```python
from build123d import *

# Parameters (mm, degrees)
BOSS_EXTRUDE1_DEPTH = 2
BOSS_EXTRUDE2_DEPTH = 19
SKETCH6_R           = 1.5
CUT_EXTRUDE1_DEPTH  = 221.788733523


with BuildPart() as part:
    # Sketch1 → Boss-Extrude1 (new body)
    with BuildSketch(Plane.XY):
        Polygon((12.5, -110.17766953), (-12.5, -110.17766953), (-30.17766953, -92.5), (-129.82233047, -92.5), (-147.5, -110.17766953), (-172.5, -110.17766953), (-190.17766953, -92.5), (-190.17766953, -67.5), (-172.5, -49.82233047), (-172.5, 49.82233047), (-190.17766953, 67.5), (-190.17766953, 92.5), (-172.5, 110.17766953), (-147.5, 110.17766953), (-129.82233047, 92.5), (-30.17766953, 92.5), (-12.5, 110.17766953), (12.5, 110.17766953), (30.17766953, 92.5), (30.17766953, 67.5), (12.5, 49.82233047), (12.5, -49.82233047), (30.17766953, -67.5), (30.17766953, -92.5), align=None)
        Polygon((-30.17766953, -67.5), (-12.5, -49.82233047), (-12.5, 49.82233047), (-30.17766953, 67.5), (-129.82233047, 67.5), (-147.5, 49.82233047), (-147.5, -49.82233047), (-129.82233047, -67.5), align=None, mode=Mode.SUBTRACT)
    extrude(amount=BOSS_EXTRUDE1_DEPTH)

    # Sketch2 → Boss-Extrude2 (add)
    with BuildSketch(Plane(origin=(0, 0, 0), x_dir=(-1, 0, 0), z_dir=(0, 0, -1))):
        Polygon((30.17766953, -67.5), (12.5, -67.5), (12.5, -49.82233047), (9.8, -49.82233047), (9.8, -70.2), (30.17766953, -70.2), align=None)
        Polygon((12.5, -92.5), (30.17766953, -92.5), (30.17766953, -89.8), (9.8, -89.8), (9.8, -110.17766953), (12.5, -110.17766953), align=None)
        Polygon((-12.5, -92.5), (-12.5, -110.17766953), (-9.8, -110.17766953), (-9.8, -89.8), (-30.17766953, -89.8), (-30.17766953, -92.5), align=None)
        Polygon((-12.5, -67.5), (-30.17766953, -67.5), (-30.17766953, -70.2), (-9.8, -70.2), (-9.8, -49.82233047), (-12.5, -49.82233047), align=None)
        Polygon((190.17766953, -67.5), (172.5, -67.5), (172.5, -49.82233047), (169.8, -49.82233047), (169.8, -70.2), (190.17766953, -70.2), align=None)
        Polygon((172.5, -92.5), (190.17766953, -92.5), (190.17766953, -89.8), (169.8, -89.8), (169.8, -110.17766953), (172.5, -110.17766953), align=None)
        Polygon((147.5, -92.5), (147.5, -110.17766953), (150.2, -110.17766953), (150.2, -89.8), (129.82233047, -89.8), (129.82233047, -92.5), align=None)
        Polygon((147.5, -67.5), (129.82233047, -67.5), (129.82233047, -70.2), (150.2, -70.2), (150.2, -49.82233047), (147.5, -49.82233047), align=None)
        Polygon((190.17766953, 92.5), (172.5, 92.5), (172.5, 110.17766953), (169.8, 110.17766953), (169.8, 89.8), (190.17766953, 89.8), align=None)
        Polygon((172.5, 67.5), (190.17766953, 67.5), (190.17766953, 70.2), (169.8, 70.2), (169.8, 49.82233047), (172.5, 49.82233047), align=None)
        Polygon((147.5, 67.5), (147.5, 49.82233047), (150.2, 49.82233047), (150.2, 70.2), (129.82233047, 70.2), (129.82233047, 67.5), align=None)
        Polygon((147.5, 92.5), (129.82233047, 92.5), (129.82233047, 89.8), (150.2, 89.8), (150.2, 110.17766953), (147.5, 110.17766953), align=None)
        Polygon((30.17766953, 92.5), (12.5, 92.5), (12.5, 110.17766953), (9.8, 110.17766953), (9.8, 89.8), (30.17766953, 89.8), align=None)
        Polygon((12.5, 67.5), (30.17766953, 67.5), (30.17766953, 70.2), (9.8, 70.2), (9.8, 49.82233047), (12.5, 49.82233047), align=None)
        Polygon((-12.5, 67.5), (-12.5, 49.82233047), (-9.8, 49.82233047), (-9.8, 70.2), (-30.17766953, 70.2), (-30.17766953, 67.5), align=None)
        Polygon((-12.5, 92.5), (-30.17766953, 92.5), (-30.17766953, 89.8), (-9.8, 89.8), (-9.8, 110.17766953), (-12.5, 110.17766953), align=None)
    extrude(amount=BOSS_EXTRUDE2_DEPTH)

    # Sketch6 → Cut-Extrude1 (cut, through all)
    with BuildSketch(Plane.XY.offset(2)):
        with Locations((-160, 80)):
            Circle(SKETCH6_R)
        with Locations((0, 80)):
            Circle(SKETCH6_R)
        with Locations((-160, -80)):
            Circle(SKETCH6_R)
        with Locations((0, -80)):
            Circle(SKETCH6_R)
    extrude(amount=-CUT_EXTRUDE1_DEPTH, mode=Mode.SUBTRACT)


solid = part.part
```
Input: part model. Units: mm. Frame: model coordinates. A direction names the side the tool comes from. Coordinates: 2 decimals unless noted, no trailing zeros. Loops run counter-clockwise (first coordinate to the right, second up) from the corner with the lowest first, then second, coordinate; pieces in that order, holes last. Notation, with made-up numbers: M 58.5,-9.75 L 100.5,-9.75 A18 cw 100.5,8.25 Z; hole C 15,80.25 d4. An arc over 180 degrees is marked long. One line per item, written item: value.
(1) Line query: line 1 along Y through (x, z) = (-136.5, -2.25); line 2 along X through (y, z) = (-51, -4); line 3 along X through (y, z) = (-80, 0.95). Output: solid intervals per line, ascending. Write a range as from..to.
Filled in:
line 1: -92.5..-89.8, -70.2..-67.5, 67.5..70.2, 89.8..92.5
line 2: -172.5..-169.8, -150.2..-147.5, -12.5..-9.8, 9.8..12.5
line 3: -190.18..-161.5, -158.5..-1.5, 1.5..30.18
(2) Reachability of faces 3 (the flat face through (-180, -89.8, -9)), 4 (the flat face through (-147.5, -59, -9)), 5 (the flat face through (-150.2, 100, -9)), 6 (the flat face through (-21, -92.5, -9)), 7 (the flat face through (-179, 61, 0)) from +Z, -Z, +X, -X, +Y, -Y: full face, straight path, thin tool, end or side. Return the list, or none.
Filled in:
face 3: -Z, +X, -X
face 4: -Z
face 5: -Z, +Y, -Y
face 6: -Z, -Y
face 7: -Z, -X
(3) Section C-C (z = -3). Give the number of separate pieces and of enclosed holes in the cut face, and give its area (3 significant figures).
Filled in:
separate pieces: 16
enclosed holes: 0
area: 1,640 mm^2
(4) Pin query (flat end, axial travel): pin 1 (9 mm diameter, centred on y = -101, z = -14, fed in from +X); pin 2 (9 mm diameter, centred on x = -137, z = -6, fed in from +Y); pin 3 (2.5 mm diameter, centred on x = -160, y = -80, fed in from +Z); pin 4 (4 mm diameter, centred on y = 1, z = -0.5, fed in from -X). Return the tip coordinate at first contact, or that it passes through.
Filled in:
pin 1: x = 12.5
pin 2: y = 92.5
pin 3: through
pin 4: x = -172.5
(5) Section D-D (x = -17). Output: boundary loops of the cut face in (y, z).
Filled in:
outline: M -105.68,0 L -92.5,0 L -92.5,-19 L -89.8,-19 L -89.8,0 L -70.2,0 L -70.2,-19 L -67.5,-19 L -67.5,0 L -54.32,0 L -54.32,2 L -105.68,2 Z; M 54.32,0 L 67.5,0 L 67.5,-19 L 70.2,-19 L 70.2,0 L 89.8,0 L 89.8,-19 L 92.5,-19 L 92.5,0 L 105.68,0 L 105.68,2 L 54.32,2 Z
(6) Section B-B (y = -17). Output: boundary loops of the cut face in (x, z).
Filled in:
outline: M -172.5,0 L -147.5,0 L -147.5,2 L -172.5,2 Z; M -12.5,0 L 12.5,0 L 12.5,2 L -12.5,2 Z
(7) Pull-direction query (X, two-part tool) for faces 1 (the flat face through (-150.2, -100, -9)), 2 (the flat face through (-181, -92.5, -9)); classes: +X half, -X half, draft (parallel to the pull), parting line (faces both ways), or undercut.
Filled in:
face 1: undercut
face 2: draft
(8) Section A-A (x = -116). Output: boundary loops of the cut face in (y, z).
Filled in:
outline: M -92.5,0 L -67.5,0 L -67.5,2 L -92.5,2 Z; M 67.5,0 L 92.5,0 L 92.5,2 L 67.5,2 Z
